Here's how the part is built. I have some questions about the finished solid (model axes, mm). A direction names the side the tool comes from. Give positions to 0.01 mm unless a question says otherwise; leave off trailing zeros. Write each loop counter-clockwise with the first axis right and the second up, starting at its lowest first coordinate (ties: lowest second). Pieces come first, ordered by that corner, then holes. Notation, with made-up numbers: (26.5, -29) - (54.5, -29) arc R37 cw to (54.5, 9) - close; hole circle Ø3 at (52.5, 87.25). An arc over 180 degrees is marked (long way). One line per item, written item: value. Start each with the question number.
1) Imagine slicing it at C-C on z = 67. Write out the boundary of the cut face in (x, y), plus the area to 3 significant figures.
2) Imagine slicing it at D-D on x = 47.5. Write out the boundary of the cut face in (y, z).
3) On a 3-axis mill with a long thin cutter (end or side, diameter ignored), from which of +Z, -Z, +X, -X, +Y, -Y can I reach the whole of each face in a straight line? I mean faces 1 (the cylindrical face through (59.93, -0.96, 23.14)), 2 (the conical face through (34.094, -1.92, 12.175)), 3 (the flat face through (46, -8, 20)). Say none if no direction works.
4) I'm going to push flat-ended pins straight in: P1, Ø4, axis at y = -1.945, z = 20, coming from the +X side; P2, Ø2, axis at x = 36, y = -2.5, coming from the +Z side; P3, Ø2, axis at x = 52, z = 30.5, coming from the -Y side. Where does each tip first touch, or does it pass through?
5) Imagine slicing it at B-B on y = 8.25. Write out the boundary of the cut face in (x, z) (3 decimals), plus the area to 3 significant figures.
6) We'd pull the mould along X, two halves only. Please class faces 4 (the conical face through (53.366, -1.773, 19.455)), 5 (the flat face through (45.91, 2.48, 37.61)), 6 (the flat face through (34.811, -5.189, 38.754)): +X half, -X half, draft (parallel to the pull), parting line (faces both ways), or undercut.
7) Imagine slicing it at A-A on x = 42.5. Write out the boundary of the cut face in (y, z).
8) Please list where these lines run through material, in increasing order: L1, parallel to Y at x = 62, z = 20 (3 decimals); L2, parallel to Z at x = 20, y = 5.25; L3, parallel to Z at x = 34.5, y = 1.75. Write a range as [from, to].
from build123d import *

# Parameters (mm, degrees)
ESBO_O1_W                                      = 130
ESBO_O1_H                                      = 20
RESSALTO_EXTRUS_O1_DEPTH                       = 95
CORTE_EXTRUS_O2_REACH                          = 22
CORTE_EXTRUS_O3_DEPTH                          = 1
CORTE_EXTRUS_O3_DEPTH_BACK                     = 61
BROCA_DE_ROSQUEAR_DE_CANO_PARA_TARRAXA_D_D     = 6.579997
BROCA_DE_ROSQUEAR_DE_CANO_PARA_TARRAXA_D_DEPTH = 10
BROCA_DE_ROSQUEAR_DE_CANO_PARA_TARRAXA_D_TIP   = 1.976830535
BROCA_DE_ROSQUEAR_DE_CANO_PARA_TARRA_2_D       = 6.579997
BROCA_DE_ROSQUEAR_DE_CANO_PARA_TARRA_2_DEPTH   = 10
BROCA_DE_ROSQUEAR_DE_CANO_PARA_TARRA_2_TIP     = 1.976830535
ESBO_O12_W                                     = 50
ESBO_O12_H                                     = 2
CORTE_EXTRUS_O4_DEPTH                          = 40
CORTE_EXTRUS_O5_DEPTH                          = 20.611613514


with BuildPart() as part:
    # Esboço1 → Ressalto-extrusão1 (new body)
    with BuildSketch(Plane.XY):
        Rectangle(ESBO_O1_W, ESBO_O1_H)
    extrude(amount=RESSALTO_EXTRUS_O1_DEPTH)

    # Esboço2 → Corte-extrusão2 (cut, up to next)
    with BuildSketch(Plane(origin=(0, 10, 0), x_dir=(1, 0, 0), z_dir=(0, 1, 0)), mode=Mode.PRIVATE) as corte_extrus_o2_sk1:
        Polygon((15, 0), (-65, 0), (-65, -95), (5, -95), (5, -41), (35, -41), (35, -40), align=None)
    corte_extrus_o2_tool1 = extrude(corte_extrus_o2_sk1.sketch, amount=-CORTE_EXTRUS_O2_REACH, mode=Mode.PRIVATE) & part.part
    add(corte_extrus_o2_tool1.solids().sort_by_distance((-24.897504, 10, 44.887255))[0], mode=Mode.SUBTRACT)

    # Esboço3 → Corte-extrusão3 (cut, two sides)
    with BuildSketch(Plane(origin=(65, 0, 0), x_dir=(0, 0, -1), z_dir=(1, 0, 0))) as corte_extrus_o3_sk:
        Polygon((200.200134404, 50.040026881), (0, 10), (-95, -9), (-295.200134404, -49.040026881), (-375.280188165, 351.360241926), (120.120080642, 450.440295688), align=None)
    extrude(amount=CORTE_EXTRUS_O3_DEPTH, mode=Mode.SUBTRACT)
    extrude(corte_extrus_o3_sk.sketch, amount=-CORTE_EXTRUS_O3_DEPTH_BACK, mode=Mode.SUBTRACT)

    # Broca de rosquear de cano para tarraxa d
    with Locations(Plane(origin=(65, 0, 0), x_dir=(0, 0, -1), z_dir=(1, 0, 0))):
        with Locations((-20, -1.945)):
            Hole(BROCA_DE_ROSQUEAR_DE_CANO_PARA_TARRAXA_D_D / 2, depth=BROCA_DE_ROSQUEAR_DE_CANO_PARA_TARRAXA_D_DEPTH)
            with Locations((0, 0, -(BROCA_DE_ROSQUEAR_DE_CANO_PARA_TARRAXA_D_DEPTH + BROCA_DE_ROSQUEAR_DE_CANO_PARA_TARRAXA_D_TIP / 2))):  # 118° drill point
                Cone(0, BROCA_DE_ROSQUEAR_DE_CANO_PARA_TARRAXA_D_D / 2, BROCA_DE_ROSQUEAR_DE_CANO_PARA_TARRAXA_D_TIP, mode=Mode.SUBTRACT)

    # Broca de rosquear de cano para tarra 2
    with Locations(Plane(origin=(12, 0, -6), x_dir=(0.447213595, 0, 0.894427191), z_dir=(-0.894427191, 0, 0.447213595))):
        with Locations((26.708203932, -1.945)):
            Hole(BROCA_DE_ROSQUEAR_DE_CANO_PARA_TARRA_2_D / 2, depth=BROCA_DE_ROSQUEAR_DE_CANO_PARA_TARRA_2_DEPTH)
            with Locations((0, 0, -(BROCA_DE_ROSQUEAR_DE_CANO_PARA_TARRA_2_DEPTH + BROCA_DE_ROSQUEAR_DE_CANO_PARA_TARRA_2_TIP / 2))):  # 118° drill point
                Cone(0, BROCA_DE_ROSQUEAR_DE_CANO_PARA_TARRA_2_D / 2, BROCA_DE_ROSQUEAR_DE_CANO_PARA_TARRA_2_TIP, mode=Mode.SUBTRACT)

    # Esboço12 → Corte-extrusão4 (cut)
    with BuildSketch(Plane(origin=(0, 0, 0), x_dir=(-1, 0, 0), z_dir=(0, 0, -1))):
        with Locations((-40, -9)):
            Rectangle(ESBO_O12_W, ESBO_O12_H)
    extrude(amount=-CORTE_EXTRUS_O4_DEPTH, mode=Mode.SUBTRACT)

    # Esboço13 → Corte-extrusão5 (cut, through all)
    with BuildSketch(Plane(origin=(0, 9.615384615, 1.923076923), x_dir=(1, 0, 0), z_dir=(0, 0.980580676, 0.196116135))):
        Polygon((35, -38.830994757), (65, -94.920209407), (66.558450481, -100.096318767), (-6.379545029, -94.920209407), (-1.820755469, -30.681038758), (34.269484804, -39.561509954), align=None)
    extrude(amount=-CORTE_EXTRUS_O5_DEPTH, mode=Mode.SUBTRACT)


solid = part.part
Numbers:
1. outline: (49.73, -3.4) - (50.42, -10) - (65, -10) - (65, -3.4) - close
1. area: 98.5 mm^2
2. outline: (-10, 40) - (-8, 40) - (-8, 0) - (10, 0) - (-2.58, 62.92) - (-10, 61.43) - close
3. face 1: +X
3. face 2: none
3. face 3: -Z, +X, -X, -Y
4. P1: x = 54.22
4. P2: z = 42.92
4. P3: y = -8
5. outline: (15, 0) - (65, 0) - (65, 8.75) - (19.375, 8.75) - close
5. area: 418 mm^2
6. face 4: +X half
6. face 5: draft
6. face 6: undercut
7. outline: (-10, 40) - (-8, 40) - (-8, 0) - (10, 0) - (-0.75, 53.75) - (-10, 51.9) - close
8. L1: [-8, -5.235], [1.345, 6]
8. L2: [0, 10]
8. L3: [0, 39]
